```python
from build123d import *

# Parameters (mm, degrees)
CROQUIS1_W               = 20.7
CROQUIS1_H               = 41.4
SALIENTE_EXTRUIR1_DEPTH  = 2.78
CHAFL_N1_SIZE            = 1.6
CROQUIS4_R               = 0.8
CORTAR_EXTRUIR2_DEPTH    = 0.2
REDONDEO5_R              = 1.2
CORTAR_EXTRUIR5_DEPTH    = 1.6
CHAFL_N2_SIZE            = 0.2
CROQUIS10_R              = 1.5
SALIENTE_EXTRUIR2_DEPTH  = 1.5
REDONDEO6_R              = 0.3
REDONDEO6_OF_SIMETR_A1_R = 0.3


# Read off the part's stored shape, not the designer's step: Simetría4
with BuildPart() as part:
    # Croquis1 → Saliente-Extruir1 (new body)
    with BuildSketch(Plane(origin=(0, 0, 0), x_dir=(1, 0, 0), z_dir=(0, 1, 0))):
        Rectangle(CROQUIS1_W, CROQUIS1_H)
    extrude(amount=SALIENTE_EXTRUIR1_DEPTH)

    # Chaflán1
    chafl_n1_edges = [part.edges().sort_by_distance(p)[0] for p in [
        (-10.35, 2.78, 0),
        (0, 2.78, 20.7),
        (10.35, 2.78, 0),
        (0, 2.78, -20.7),
    ]]
    chamfer(chafl_n1_edges, length=CHAFL_N1_SIZE)

    # Croquis4 → Cortar-Extruir2 (cut)
    with BuildSketch(Plane(origin=(0, 2.78, 0), x_dir=(1, 0, 0), z_dir=(0, 1, 0))):
        with Locations(Location((0, 0, 0), (0, 0, 270))):
            Circle(CROQUIS4_R)
    extrude(amount=-CORTAR_EXTRUIR2_DEPTH, mode=Mode.SUBTRACT)

    # Redondeo5
    redondeo5_edges = [part.edges().sort_by_distance(p)[0] for p in [
        (10.35, 0.59, 20.7),
        (-10.35, 0.59, 20.7),
        (-10.35, 0.59, -20.7),
        (10.35, 0.59, -20.7),
    ]]
    fillet(redondeo5_edges, radius=REDONDEO5_R)

    # Croquis8 → Cortar-Extruir5 (cut)
    with BuildSketch(Plane(origin=(0, 2.78, 0), x_dir=(1, 0, 0), z_dir=(0, 1, 0))):
        with BuildLine():
            Line((-10.35, -20.7), (-6.55, -20.7))
            Line((-6.55, -20.7), (-6.55, -18.1))
            ThreePointArc((-6.55, -18.1), (-6.901471863, -17.251471863), (-7.75, -16.9))
            Line((-7.75, -16.9), (-10.35, -16.9))
            Line((-10.35, -16.9), (-10.35, -20.7))
        make_face()
        with BuildLine():
            Line((6.55, -20.7), (6.55, -18.1))
            ThreePointArc((6.55, -18.1), (6.901471863, -17.251471863), (7.75, -16.9))
            Line((7.75, -16.9), (10.35, -16.9))
            Line((10.35, -16.9), (10.35, -20.7))
            Line((10.35, -20.7), (6.55, -20.7))
        make_face()
        with BuildLine():
            Line((10.35, 20.7), (6.55, 20.7))
            Line((6.55, 20.7), (6.55, 18.1))
            ThreePointArc((6.55, 18.1), (6.901471863, 17.251471863), (7.75, 16.9))
            Line((7.75, 16.9), (10.35, 16.9))
            Line((10.35, 16.9), (10.35, 20.7))
        make_face()
        with BuildLine():
            Line((-6.55, 20.7), (-6.55, 18.1))
            ThreePointArc((-6.55, 18.1), (-6.901471863, 17.251471863), (-7.75, 16.9))
            Line((-7.75, 16.9), (-10.35, 16.9))
            Line((-10.35, 16.9), (-10.35, 20.7))
            Line((-10.35, 20.7), (-6.55, 20.7))
        make_face()
    extrude(amount=-CORTAR_EXTRUIR5_DEPTH, mode=Mode.SUBTRACT)

    # Chaflán2
    # the kernel refuses this chamfer: 0.2 mm, written as the material it takes off along each edge
    with BuildSketch(Plane(origin=(9.15, 1.18, -19.5), x_dir=(1, 0, 0), z_dir=(0, 0, 1))) as chafl_n2_piece_1:
        Polygon((1.2, -CHAFL_N2_SIZE), (1.2 - CHAFL_N2_SIZE, 0), (1.2, 0), align=None)
    revolve(axis=Axis((9.15, 1.18, -19.5), (0, 1, 0)), revolution_arc=90, mode=Mode.SUBTRACT)
    with BuildSketch(Plane(origin=(9.15, 1.18, -20.7), x_dir=(0, -0.999621916911297, -0.027495876610578732), z_dir=(-1, 0, 0)), Plane(origin=(-10.35, 1.18, -19.5), x_dir=(-0.02749587661058736, -0.9996219169112966, 0), z_dir=(0, 0, 1)), Plane(origin=(-6.55, 1.18, -20.7), x_dir=(0, -0.999621916911297, -0.027495876610578732), z_dir=(-1, 0, 0)), Plane(origin=(10.35, 1.18, -16.9), x_dir=(0.02749587661058736, -0.9996219169112966, 0), z_dir=(0, 0, -1)), Plane(origin=(6.55, 1.18, 20.7), x_dir=(0, -0.999621916911297, 0.027495876610578732), z_dir=(1, 0, 0)), Plane(origin=(-9.15, 1.18, 20.7), x_dir=(0, -0.999621916911297, 0.027495876610578732), z_dir=(1, 0, 0))) as chafl_n2_piece_2:
        Polygon((CHAFL_N2_SIZE * 0.999621916911, CHAFL_N2_SIZE * 0.0274958766106), (-CHAFL_N2_SIZE * 0.0274958766106, CHAFL_N2_SIZE * 0.999621916911), (0, 0), align=None)
    extrude(amount=2.6, mode=Mode.SUBTRACT)
    with BuildSketch(Plane(origin=(-9.15, 1.18, -19.5), x_dir=(0, 0, -1), z_dir=(1, 0, 0))) as chafl_n2_piece_3:
        Polygon((1.2, -CHAFL_N2_SIZE), (1.2 - CHAFL_N2_SIZE, 0), (1.2, 0), align=None)
    revolve(axis=Axis((-9.15, 1.18, -19.5), (0, 1, 0)), revolution_arc=90, mode=Mode.SUBTRACT)
    with BuildSketch(Plane(origin=(-10.35, 1.18, 16.9), x_dir=(0.9996219169112966, 0.02749587661058634, 0), z_dir=(0, 0, 1)), Plane(origin=(10.35, 1.18, 19.5), x_dir=(-0.9996219169112966, 0.02749587661058634, 0), z_dir=(0, 0, -1))) as chafl_n2_piece_4:
        Polygon((CHAFL_N2_SIZE * 0.999621916911, -CHAFL_N2_SIZE * 0.0274958766106), (-CHAFL_N2_SIZE * 0.0274958766106, -CHAFL_N2_SIZE * 0.999621916911), (0, 0), align=None)
    extrude(amount=2.6, mode=Mode.SUBTRACT)
    with BuildSketch(Plane(origin=(-9.15, 1.18, 19.5), x_dir=(-1, 0, 0), z_dir=(0, 0, -1))) as chafl_n2_piece_5:
        Polygon((1.2 - CHAFL_N2_SIZE, 0), (1.2, -CHAFL_N2_SIZE), (1.2, 0), align=None)
    revolve(axis=Axis((-9.15, 1.18, 19.5), (0, 1, 0)), revolution_arc=90, mode=Mode.SUBTRACT)
    with BuildSketch(Plane(origin=(9.15, 1.18, 19.5), x_dir=(0, 0, 1), z_dir=(-1, 0, 0))) as chafl_n2_piece_6:
        Polygon((1.2 - CHAFL_N2_SIZE, 0), (1.2, -CHAFL_N2_SIZE), (1.2, 0), align=None)
    revolve(axis=Axis((9.15, 1.18, 19.5), (0, 1, 0)), revolution_arc=90, mode=Mode.SUBTRACT)

    # Croquis10 → Saliente-Extruir2 (add)
    with BuildSketch(Plane(origin=(0, 1.18, 0), x_dir=(1, 0, 0), z_dir=(0, 1, 0))):
        with Locations(Location((-8.35, -18.7, 0), (0, 0, 90))):
            Circle(CROQUIS10_R)
    saliente_extruir2 = extrude(amount=SALIENTE_EXTRUIR2_DEPTH)

    # Redondeo6
    redondeo6_edges = [part.edges().sort_by_distance(p)[0] for p in [
        (-8.35, 2.68, 20.2),
    ]]
    fillet(redondeo6_edges, radius=REDONDEO6_R)

    # Simetría1: Saliente-Extruir2 across plane
    add(saliente_extruir2.mirror(Plane(origin=(0, 0, 0), x_dir=(0, 0, 1), z_dir=(1, 0, 0))))

    # Redondeo6 of Simetría1
    redondeo6_of_simetr_a1_edges = [part.edges().sort_by_distance(p)[0] for p in [
        (8.35, 2.68, 20.2),
    ]]
    fillet(redondeo6_of_simetr_a1_edges, radius=REDONDEO6_OF_SIMETR_A1_R)

    # Simetría4 outline → Simetría4 (revolve)
    with BuildSketch(Plane(origin=(8.35, 0, -18.7), x_dir=(1, 0, 0), z_dir=(0, 0, 1))):
        with BuildLine():
            Line((1.2, 2.68), (0, 2.68))
            Line((0, 2.68), (0, 1.18))
            Line((0, 1.18), (1.5, 1.18))
            Line((1.5, 1.18), (1.5, 2.38))
            ThreePointArc((1.5, 2.38), (1.412132034, 2.592132034), (1.2, 2.68))
        make_face()
    revolve(axis=Axis((8.35, 0, -18.7), (0, 1, 0)))

    # Simetr_a4 2 outline → Simetr_a4 2 (revolve)
    with BuildSketch(Plane(origin=(-8.35, 0, -18.7), x_dir=(1, 0, 0), z_dir=(0, 0, 1))):
        with BuildLine():
            Line((1.2, 2.68), (0, 2.68))
            Line((0, 2.68), (0, 1.18))
            Line((0, 1.18), (1.5, 1.18))
            Line((1.5, 1.18), (1.5, 2.38))
            ThreePointArc((1.5, 2.38), (1.412132034, 2.592132034), (1.2, 2.68))
        make_face()
    revolve(axis=Axis((-8.35, 0, -18.7), (0, 1, 0)))


solid = part.part
```
CAD build for the part. Positions are in the model's coordinates, mm. A direction names the side the tool comes from. Give positions to 0.01 mm unless a question says otherwise; leave off trailing zeros. Order: outer loops, then holes, each group sorted by start corner. A loop starts at its lowest first (then second) coordinate and runs counter-clockwise, first axis right, second up. Notation, with made-up numbers: M 48,45.5 L 86,45.5 A21 ccw 86,79.5 Z; hole C 50,28 d7. An arc over 180 degrees is marked long. Put each result on its own line as item: value. Start each with the question number.
(1) Saw through at B-B, the plane z = -18.7. Write the cut outline in (x, y).
(2) Saw through at D-D, the plane x = 0. Write the cut outline in (y, z).
(3) Flat gauge pins, fed straight in: pin 1 Ø0.9 at (y, z) = (2, 20) entering from -X; pin 2 Ø1.9 at (x, z) = (8.5, -18.5) entering from +Y; pin 3 Ø1.5 at (x, y) = (4, 2) entering from -Z. Where does each tip first touch, or does it go through?
(4) Saw through at A-A, the plane x = -8.35. Write the cut outline in (y, z).
(5) Drill centre lines: line 1 along Z through (x, y) = (-7.75, 1.55); line 2 along X through (y, z) = (1.75, -19); line 3 along X through (y, z) = (2.7, 0). Where is each one in solid material? Low to high.
(6) Which spindle directions (+Z, -Z, +X, -X, +Y, -Y) get a long thin tool onto all of the face, cutting with end or side? Do faces 1 (the cylindrical face through (9.837, 1.772, 18.895)), 2 (the flat face through (9, 2, 16.9)), 3 (the flat face through (-9, 2, 16.9)), 4 (the flat face through (6.55, 2, 19)). Say none if no direction does.
(7) Mould opens along X. For faces 5 (the flat face through (0, 0, 0)), 6 (the flat face through (10.35, 1, 0)), 7 (the cylindrical face through (-9.837, 1.772, 18.895)), 8 (the flat face through (-0.09, 1.99, 19.89)) say: +X half, -X half, draft (parallel to the pull), parting line (faces both ways), or undercut.
(8) Saw through at C-C, the plane z = 0. Write the cut outline in (x, y).
Check result:
1. outline: M -10.35,0 L 10.35,0 L 10.35,0.98 L 10.15,1.18 L 9.85,1.18 L 9.85,2.38 A0.3 ccw 9.55,2.68 L 7.15,2.68 A0.3 ccw 6.85,2.38 L 6.85,1.18 L 6.55,1.18 L 6.55,2.78 L -6.55,2.78 L -6.55,1.18 L -6.85,1.18 L -6.85,2.38 A0.3 ccw -7.15,2.68 L -9.55,2.68 A0.3 ccw -9.85,2.38 L -9.85,1.18 L -10.15,1.18 L -10.35,0.98 Z
2. outline: M 0,-20.7 L 1.18,-20.7 L 2.78,-19.1 L 2.78,-0.8 L 2.58,-0.8 L 2.58,0.8 L 2.78,0.8 L 2.78,19.1 L 1.18,20.7 L 0,20.7 Z
3. pin 1: stops at x = -9.59
3. pin 2: stops at y = 2.68
3. pin 3: stops at z = -20.63
4. outline: M 0,-20.7 L 0.98,-20.7 L 1.18,-20.5 L 1.18,-20.2 L 2.38,-20.2 A0.3 ccw 2.68,-19.9 L 2.68,-17.5 A0.3 ccw 2.38,-17.2 L 1.18,-17.2 L 1.18,-16.9 L 2.78,-16.9 L 2.78,16.9 L 1.18,16.9 L 1.18,17.2 L 2.38,17.2 A0.3 ccw 2.68,17.5 L 2.68,19.9 A0.3 ccw 2.38,20.2 L 1.18,20.2 L 1.18,20.5 L 0.98,20.7 L 0,20.7 Z
5. line 1: z = -20.07 to -17.33, -16.9 to 16.9, 17.33 to 20.07
5. line 2: x = -9.82 to -6.88, -6.55 to 6.55, 6.88 to 9.82
5. line 3: x = -8.83 to -0.8, 0.8 to 8.83
6. face 1: +Y
6. face 2: +X, +Y
6. face 3: -X, +Y
6. face 4: +Z, +Y
7. face 5: draft
7. face 6: +X half
7. face 7: undercut
7. face 8: undercut
8. outline: M -10.35,0 L 10.35,0 L 10.35,1.18 L 8.75,2.78 L 0.8,2.78 L 0.8,2.58 L -0.8,2.58 L -0.8,2.78 L -8.75,2.78 L -10.35,1.18 Z
